Autodesk Inventor part; units mm, degrees
ref_plane "YZ Plane" through (0, 0, 0) normal (1, 0, 0) x (0, 1, 0)
ref_plane "XZ Plane" through (0, 0, 0) normal (0, 1, 0) x (-1, 0, 0)
ref_plane "XY Plane" through (0, 0, 0) normal (0, 0, 1) x (1, 0, 0)
sketch "Sketch1" plane through (0, 0, 0) normal (0, 1, 0) x (-1, 0, 0)
  line L0 (-73, 65) -> (73, 65)
  line L1 (73, 65) -> (73, -65)
  line L2 (73, -65) -> (-73, -65)
  line L3 (-73, -65) -> (-73, 65)
  line L4 (-73, 65) -> (73, -65) construction
  line L5 (73, 65) -> (-73, -65) construction
  point P0 (0, 0)
  dimension "d0" = 146
  dimension "d1" = 130
extrude "Extrusion1" add sketch "Sketch1" along normal blind 115
sketch "Sketch2" plane through (0, 0, 0) normal (0, -1, 0) x (1, 0, 0)
  line L0 (-69.125, -61.125) -> (69.125, -61.125)
  line L1 (69.125, -61.125) -> (69.125, 61.125)
  line L2 (69.125, 61.125) -> (-69.125, 61.125)
  line L3 (-69.125, 61.125) -> (-69.125, -61.125)
  line L4 (-69.125, -61.125) -> (69.125, 61.125) construction
  line L5 (69.125, -61.125) -> (-69.125, 61.125) construction
  line L6 (-69.125, 61.125) -> (69.125, 61.125)
  line L7 (69.125, 61.125) -> (69.125, 91.125)
  line L8 (69.125, 91.125) -> (-69.125, 91.125)
  line L9 (-69.125, 91.125) -> (-69.125, 61.125)
  point P0 (0, 0)
  dimension "d4" = 138.25
  dimension "d5" = 122.25
  dimension "d6" = 138.25
  dimension "d7" = 30
extrude "Extrusion2" cut sketch "Sketch2" against normal through all
sketch "Sketch3" plane through (0, 115, 0) normal (0, 1, 0) x (1, 0, 0)
  line L0 (-69.125, 61.125) -> (69.125, 61.125)
  line L1 (69.125, 61.125) -> (69.125, -65)
  line L2 (-69.125, 61.125) -> (69.125, 61.125)
  line L3 (69.125, 61.125) -> (69.125, -65)
  line L4 (69.125, -65) -> (-69.125, -65)
  line L5 (-69.125, -65) -> (-69.125, 61.125)
  line L6 (-65.125, -57.125) -> (65.125, -57.125)
  line L7 (65.125, -57.125) -> (65.125, 57.125)
  line L8 (65.125, 57.125) -> (-65.125, 57.125)
  line L9 (-65.125, 57.125) -> (-65.125, -57.125)
  line L10 (-65.125, -57.125) -> (65.125, 57.125) construction
  line L11 (65.125, -57.125) -> (-65.125, 57.125) construction
  line L12 (65.125, -57.125) -> (65.125, -65)
  line L13 (-65.125, -57.125) -> (-65.125, -65)
  point P0 (0, 0)
  dimension "d10" = 4
  dimension "d11" = 4
extrude "Extrusion3" add sketch "Sketch3" against normal blind 5 contours L0 L1 L4 L12 L7 L8 L9 L13 L5
properties part number "Cylinder Galvo Housing"
Could you check a few things on this model? Use its own coordinates, in mm. A direction names the side the tool comes from. Give positions to 0.01 mm unless a question says otherwise; leave off trailing zeros. Loops run counter-clockwise (first coordinate to the right, second up) from the corner with the lowest first, then second, coordinate; pieces in that order, holes last. Notation, with made-up numbers: (44.25, -25) - (56.25, -25) arc R20 ccw to (56.25, -15) - close; hole circle Ø9 at (77, 32). An arc over 180 degrees is marked (long way). Answer in a Markdown table with one row per item. Add a question column.
Q1. If we section it at B-B (y = 58): List the corners of the cut face in (x, z) for me (3 decimals), plus the area to 3 significant figures.
Q2. Which directions (+Z, -Z, +X, -X, +Y, -Y) give clear straight access to the entire face, cutting with the end or side of a thin tool? Please do faces 5 (the face through (65.125, 113, 3)), 6 (the face through (-69.125, 54, 3)), 7 (the face through (0, 0, -62)).
Q3. We'd pull the mould along X, two halves only. Please class faces 1 (the face through (-1, 57, -65)), 2 (the face through (73, 57, -1)), 3 (the face through (1, 113, -57.125)), 4 (the face through (69.125, 54, 1)): +X half, -X half, draft (parallel to the pull), parting line (faces both ways), or undercut.
Q4. Please list where these lines run through material, in increasing order: L1, parallel to X at y = 53.5, z = -13.5 (3 decimals); L2, parallel to Z at x = -7.5, y = 41 (3 decimals); L3, parallel to Y at x = 66.5, z = 54. Write a range as from..to.
Q5. If we section it at A-A (z = 1): List the corners of the cut face in (x, y) for me (3 decimals), plus the area to 3 significant figures.
Q6. If we section it at C-C (x = -36): List the corners of the cut face in (y, z) for me (3 decimals).
Q7. For pin 1 (2.5 mm diameter, centred on x = 5.5, y = 111.5, fed in from +Z) (3 decimals), with a flat end and sliding along its axis, tell me the tip position at first contact or that it passes through.
The answers:
| question | item | result |
|---|---|---|
| 1 | outline | (-73, -65) - (73, -65) - (73, 65) - (69.125, 65) - (69.125, -61.125) - (-69.125, -61.125) - (-69.125, 65) - (-73, 65) - close |
| 1 | area | 1,540 mm^2 |
| 2 | face 5 | +Z, +Y, -Y |
| 2 | face 6 | +Z, -Y |
| 2 | face 7 | +Z, -Z, +X, -X, -Y |
| 3 | face 1 | draft |
| 3 | face 2 | +X half |
| 3 | face 3 | undercut |
| 3 | face 4 | undercut |
| 4 | L1 | x = -73..-69.125, 69.125..73 |
| 4 | L2 | z = -65..-61.125 |
| 4 | L3 | y = 110..115 |
| 5 | outline | (-73, 0) - (-69.125, 0) - (-69.125, 110) - (-65.125, 110) - (-65.125, 115) - (-73, 115) - close; (65.125, 110) - (69.125, 110) - (69.125, 0) - (73, 0) - (73, 115) - (65.125, 115) - close |
| 5 | area | 931 mm^2 |
| 6 | outline | (0, -65) - (115, -65) - (115, -57.125) - (110, -57.125) - (110, -61.125) - (0, -61.125) - close |
| 7 | pin 1 | stops at z = -57.125 |
